Source: CAD feature listing. Evaluate the final solid. Frame: model axes, mm. A direction names the side the tool comes from. Round coordinates to 2 decimals unless told otherwise and drop trailing zeros. Order: outer loops, then holes, each group sorted by start corner. A loop starts at its lowest first (then second) coordinate and runs counter-clockwise, first axis right, second up. Notation, with made-up numbers: (3.25, -6) - (29.25, -6) arc R25 ccw to (29.25, 33) - close; hole circle Ø9 at (45, 35). An arc over 180 degrees is marked (long way). Use one line per item in the form item = value. Start each with the question number.
Q1. Ray query, line 1 (Z direction, x = -57.5, y = 9.25); line 2 (X direction, y = 5.25, z = 57.15); line 3 (X direction, y = -0.25, z = -63.5). Return the intervals inside material, ascending. Write a range as [from, to].
Q2. Draft query along X for faces 5 (the flat face through (-54.098, 19, 83)), 6 (the flat face through (53.15, 4, -1)), 7 (the flat face through (-57, 8, 1)), 8 (the flat face through (41, 17.05, -79)). Return one class per face: released by +X, released by -X, zero draft, split by the parting line, or undercut.
Q3. Cut plane B-B, the plane x = -18. Return the cut outline in (y, z).
Q4. Cut plane C-C, the plane y = 5.5. Give the number of separate pieces and of enclosed holes in the cut face, and give its area (3 significant figures).
Q5. Cut plane A-A, the plane z = 45. Return the cut outline in (x, y).
Q6. Set-up query: faces 1 (the flat face through (41.734, 5.448, -63.204)), 2 (the flat face through (-37.263, 19.022, -87.737)), 3 (the flat face through (27, 19, 72.2)), 4 (the flat face through (-61, 10, -57)). Return all of +Z, -Z, +X, -X, +Y, -Y with unobstructed straight access to the full face (end or side cutting, diameter ignored); none if empty.
Q7. Pin query (flat end, axial travel): pin 1 Ø17.5 at (x, z) = (54.5, 56.5) entering from +Y; pin 2 Ø6.5 at (x, y) = (26, 14) entering from -Z; pin 3 Ø1 at (y, z) = (15.5, 57.5) entering from -X; pin 4 Ø1.5 at (x, y) = (44.5, 9) entering from -Z. Return the tip coordinate at first contact, or that it passes through.
from build123d import *

# Parameters (mm, degrees)
BOSS_EXTRUDE1_DEPTH            = 8
BOSS_EXTRUDE2_DEPTH            = 2
BOSS_EXTRUDE3_DEPTH            = 9.05
SKETCH4_R                      = 2.25
BOSS_EXTRUDE4_DEPTH            = 4
CUT_EXTRUDE1_REACH             = 89.395
SKETCH5_W                      = 12.364675298
SKETCH5_H                      = 8
CUT_EXTRUDE1_DIRECTION_2_DEPTH = 88.395228364
CUT_EXTRUDE2_DEPTH             = 9.171573
CUT_EXTRUDE3_REACH             = 115.505
SKETCH8_W                      = 3.39411255
SKETCH8_H                      = 9.05
CUT_EXTRUDE3_DIRECTION_2_REACH = 115.505
BOSS_EXTRUDE5_DEPTH            = 16.456854
CUT_EXTRUDE4_DEPTH             = 114.504844196
SKETCH12_R                     = 3.6
CUT_EXTRUDE5_DEPTH             = 114.645358602
BOSS_EXTRUDE6_START            = 2
SKETCH13_W                     = 16
SKETCH13_H                     = 16
SKETCH13_R                     = 3.6
BOSS_EXTRUDE6_DEPTH            = 2
CUT_EXTRUDE6_REACH             = 182.475
CUT_EXTRUDE6_DIRECTION_2_DEPTH = 15


with BuildPart() as part:
    # Sketch1 → Boss-Extrude1 (new body)
    with BuildSketch(Plane(origin=(0, 0, 0), x_dir=(1, 0, 0), z_dir=(0, 1, 0))):
        Polygon((-53.15, 0), (-61.15, 0), (-61.15, -49.15), (-65.15, -49.15), (-65.15, -65.15), (-57.635281374, -65.15), (-32.585281374, -90.2), (0, -90.2), (0, -82.2), (-20.1, -82.2), (-20.1, -77.4), (-34.071572875, -77.4), (-39.3, -72.171572875), (-39.3, -58.2), (-49.15, -58.2), (-49.15, -49.15), (-53.15, -49.15), align=None)
    extrude(amount=BOSS_EXTRUDE1_DEPTH)

    # Sketch2 → Boss-Extrude2 (add)
    with BuildSketch(Plane.XZ):
        Polygon((-49.15, 58.2), (-49.15, 49.15), (-65.15, 49.15), (-65.15, 65.15), (-49.15, 65.15), align=None)
    extrude(amount=BOSS_EXTRUDE2_DEPTH)

    # Sketch3 → Boss-Extrude3 (add)
    with BuildSketch(Plane(origin=(0, 8, 0), x_dir=(1, 0, 0), z_dir=(0, 1, 0))):
        Polygon((-39.3, -58.2), (-45.3, -58.2), (-45.3, -74.656854249), (-36.556854249, -83.4), (-20.1, -83.4), (-20.1, -77.4), (-34.071572875, -77.4), (-39.3, -72.171572875), align=None)
    extrude(amount=BOSS_EXTRUDE3_DEPTH)

    # Sketch4 → Boss-Extrude4 (add)
    with BuildSketch(Plane(origin=(0, 17.05, 0), x_dir=(1, 0, 0), z_dir=(0, 1, 0))):
        Polygon((-45.3, -58.2), (-34.1, -58.2), (-34.1, -72.2), (-20.1, -72.2), (-20.1, -83.4), (-32.925631329, -83.4), (-41.723475836, -92.197844507), (-48.972213178, -92.197844507), (-54.097844507, -87.072213178), (-54.097844507, -79.823475836), (-45.3, -71.025631329), align=None)
        with Locations(Location((-45.347844507, -83.447844507, 0), (0, 0, 270))):
            Circle(SKETCH4_R, mode=Mode.SUBTRACT)
    extrude(amount=BOSS_EXTRUDE4_DEPTH)

    # Sketch5 → Cut-Extrude1 (cut, up to next)
    with BuildSketch(Plane(origin=(-59.978427125, 0, 59.978427125), x_dir=(0.7071067811865475, 0, 0.7071067811865477), z_dir=(-0.7071067811865477, 0, 0.7071067811865475)), mode=Mode.PRIVATE) as cut_extrude1_sk1:
        with Locations((26.940768363, 13.05)):
            Rectangle(SKETCH5_W, SKETCH5_H)
    cut_extrude1_tool1 = extrude(cut_extrude1_sk1.sketch, amount=-CUT_EXTRUDE1_REACH, mode=Mode.PRIVATE) & part.part
    add(cut_extrude1_tool1.solids().sort_by_distance((-40.928427, 13.05, 79.028427))[0], mode=Mode.SUBTRACT)

    # Sketch5 → Cut-Extrude1 direction 2 (cut)
    with BuildSketch(Plane(origin=(-59.978427125, 0, 59.978427125), x_dir=(0.7071067811865475, 0, 0.7071067811865477), z_dir=(-0.7071067811865477, 0, 0.7071067811865475))):
        with Locations((26.940768363, 13.05)):
            Rectangle(SKETCH5_W, SKETCH5_H)
    extrude(amount=CUT_EXTRUDE1_DIRECTION_2_DEPTH, mode=Mode.SUBTRACT)

    # Sketch6 → Cut-Extrude2 (cut)
    with BuildSketch(Plane(origin=(-20.1, 0, 0), x_dir=(0, 0, -1), z_dir=(1, 0, 0))):
        Polygon((-82.2, 0), (-77.4, 11.05), (-77.4, 0), align=None)
    cut_extrude2 = extrude(amount=-CUT_EXTRUDE2_DEPTH, mode=Mode.SUBTRACT)

    # Mirror1: Cut-Extrude2 across plane
    add(cut_extrude2.mirror(Plane(origin=(19.05, 0, 19.05), x_dir=(-0.7071067811865477, 0, 0.7071067811865474), z_dir=(0.7071067811865476, 0, 0.7071067811865476))), mode=Mode.SUBTRACT)

    # Cut-Extrude3: up to this face of the body (flat: up to its plane)
    cut_extrude3_end = Plane(part.part.faces().sort_by_distance((-41.7, 5.525, 62.7857865))[0])
    # Sketch8 → Cut-Extrude3 (cut, up to the picked face)
    with BuildSketch(Plane(origin=(19.05, 0, 19.05), x_dir=(0.7071067811865476, 0, -0.7071067811865476), z_dir=(0.7071067811865476, 0, 0.7071067811865476)), mode=Mode.PRIVATE) as cut_extrude3_sk1:
        with Locations((-77.125248815, 4.525)):
            Rectangle(SKETCH8_W, SKETCH8_H)
    cut_extrude3_tool1 = split(extrude(cut_extrude3_sk1.sketch, amount=-CUT_EXTRUDE3_REACH, mode=Mode.PRIVATE), bisect_by=cut_extrude3_end, keep=Keep.BOTH, mode=Mode.PRIVATE)
    add(cut_extrude3_tool1.solids().sort_by(Axis((-35.485786, 4.525, 73.585786), (-0.7071067811865476, 0, -0.7071067811865476)))[0], mode=Mode.SUBTRACT)

    # Cut-Extrude3 direction 2: up to this face of the body (flat: up to its plane)
    cut_extrude3_direction_2_end = Plane(part.part.faces().sort_by_distance((-24.6857865, 5.525, 79.8))[0])
    # Sketch8 → Cut-Extrude3 direction 2 (cut, up to the picked face)
    with BuildSketch(Plane(origin=(19.05, 0, 19.05), x_dir=(0.7071067811865476, 0, -0.7071067811865476), z_dir=(0.7071067811865476, 0, 0.7071067811865476)), mode=Mode.PRIVATE) as cut_extrude3_direction_2_sk1:
        with Locations((-77.125248815, 4.525)):
            Rectangle(SKETCH8_W, SKETCH8_H)
    cut_extrude3_direction_2_tool1 = split(extrude(cut_extrude3_direction_2_sk1.sketch, amount=CUT_EXTRUDE3_DIRECTION_2_REACH, mode=Mode.PRIVATE), bisect_by=cut_extrude3_direction_2_end, keep=Keep.BOTH, mode=Mode.PRIVATE)
    add(cut_extrude3_direction_2_tool1.solids().sort_by(Axis((-35.485786, 4.525, 73.585786), (0.7071067811865476, 0, 0.7071067811865476)))[0], mode=Mode.SUBTRACT)

    # Sketch10 → Boss-Extrude5 (add)
    with BuildSketch(Plane(origin=(-20.1, 0, 0), x_dir=(0, 0, -1), z_dir=(1, 0, 0))):
        Polygon((-83.4, 12.296887645), (-85.26652133, 8), (-83.4, 8), align=None)
    boss_extrude5 = extrude(amount=-BOSS_EXTRUDE5_DEPTH)

    # Sketch11 → Cut-Extrude4 (cut, through all)
    with BuildSketch(Plane(origin=(19.05, 0, 19.05), x_dir=(0.7071067811865476, 0, -0.7071067811865476), z_dir=(0.7071067811865476, 0, 0.7071067811865476))):
        Polygon((-84.82230509, 12.296887645), (-86.142134979, 8), (-84.82230509, 8), align=None)
    cut_extrude4 = extrude(amount=CUT_EXTRUDE4_DEPTH, mode=Mode.SUBTRACT)

    # Mirror2: Boss-Extrude5, Cut-Extrude4 across plane
    add(boss_extrude5.mirror(Plane(origin=(19.05, 0, 19.05), x_dir=(-0.7071067811865477, 0, 0.7071067811865474), z_dir=(0.7071067811865476, 0, 0.7071067811865476))))
    add(cut_extrude4.mirror(Plane(origin=(19.05, 0, 19.05), x_dir=(-0.7071067811865477, 0, 0.7071067811865474), z_dir=(0.7071067811865476, 0, 0.7071067811865476))), mode=Mode.SUBTRACT)

    # Sketch12 → Cut-Extrude5 (cut, through all)
    with BuildSketch(Plane(origin=(0, 8, 0), x_dir=(1, 0, 0), z_dir=(0, 1, 0))):
        with Locations(Location((-57.15, -57.15, 0), (0, 0, 270))):
            Circle(SKETCH12_R)
    extrude(amount=-CUT_EXTRUDE5_DEPTH, mode=Mode.SUBTRACT)

    # Mirror3: part across plane


with BuildPart() as part_1:
    add(part.part)
    add(part.part.mirror(Plane(origin=(-53.15, 8, 0), x_dir=(1, 0, 0), z_dir=(0, 0, 1))))

    # Mirror4: part across plane


with BuildPart() as part_2:
    add(part_1.part)
    add(part_1.part.mirror(Plane(origin=(0, 8, -90.2), x_dir=(0, 0, 1), z_dir=(-1, 0, 0))))

    # Sketch13 → Boss-Extrude6 (add)
    # profile 1 of 4: a face of its own
    with BuildSketch(Plane(origin=(0, 8, 0), x_dir=(1, 0, 0), z_dir=(0, 1, 0)).offset(BOSS_EXTRUDE6_START)):
        with Locations((-57.15, 57.15)):
            Rectangle(SKETCH13_W, SKETCH13_H)
        with Locations(Location((-57.15, 57.15, 0), (0, 0, 90))):
            Circle(SKETCH13_R, mode=Mode.SUBTRACT)
    # profile 2 of 4: a face of its own
    with BuildSketch(Plane(origin=(0, 8, 0), x_dir=(1, 0, 0), z_dir=(0, 1, 0)).offset(BOSS_EXTRUDE6_START)):
        with Locations((-57.15, -57.15)):
            Rectangle(SKETCH13_W, SKETCH13_H)
        with Locations(Location((-57.15, -57.15, 0), (0, 0, 270))):
            Circle(SKETCH13_R, mode=Mode.SUBTRACT)
    # profile 3 of 4: a face of its own
    with BuildSketch(Plane(origin=(0, 8, 0), x_dir=(1, 0, 0), z_dir=(0, 1, 0)).offset(BOSS_EXTRUDE6_START)):
        with Locations((57.15, -57.15)):
            Rectangle(SKETCH13_W, SKETCH13_H)
        with Locations(Location((57.15, -57.15, 0), (0, 0, 270))):
            Circle(SKETCH13_R, mode=Mode.SUBTRACT)
    # profile 4 of 4: a face of its own
    with BuildSketch(Plane(origin=(0, 8, 0), x_dir=(1, 0, 0), z_dir=(0, 1, 0)).offset(BOSS_EXTRUDE6_START)):
        with Locations((57.15, 57.15)):
            Rectangle(SKETCH13_W, SKETCH13_H)
        with Locations(Location((57.15, 57.15, 0), (0, 0, 90))):
            Circle(SKETCH13_R, mode=Mode.SUBTRACT)
    extrude(amount=-BOSS_EXTRUDE6_DEPTH)

    # Cut-Extrude6: up to this face of the body (flat: up to its plane)
    cut_extrude6_end = Plane(part_2.part.faces().sort_by_distance((25.508916271, 13.892566464, 77.4))[0])
    # Sketch14 → Cut-Extrude6 (cut, up to the picked face)
    with BuildSketch(Plane(origin=(0, 0, 74.785786438), x_dir=(-1, 0, 0), z_dir=(0, 0, -1)), mode=Mode.PRIVATE) as cut_extrude6_sk1:
        with BuildLine():
            Line((-38.891815428, 9.05), (-29.271572875, 9.05))
            Line((-29.271572875, 9.05), (-29.271572875, 0))
            Line((-29.271572875, 0), (-37.428466034, 0))
            ThreePointArc((-37.428466034, 0), (-38.292196947, 4.503647029), (-38.891815428, 9.05))
        make_face()
    cut_extrude6_tool1 = split(extrude(cut_extrude6_sk1.sketch, amount=-CUT_EXTRUDE6_REACH, mode=Mode.PRIVATE), bisect_by=cut_extrude6_end, keep=Keep.BOTH, mode=Mode.PRIVATE)
    add(cut_extrude6_tool1.solids().sort_by(Axis((33.771048, 4.647825, 74.785786), (0, 0, 1)))[0], mode=Mode.SUBTRACT)

    # Sketch14 → Cut-Extrude6 direction 2 (cut)
    with BuildSketch(Plane(origin=(0, 0, 74.785786438), x_dir=(-1, 0, 0), z_dir=(0, 0, -1))):
        with BuildLine():
            Line((-38.891815428, 9.05), (-29.271572875, 9.05))
            Line((-29.271572875, 9.05), (-29.271572875, 0))
            Line((-29.271572875, 0), (-37.428466034, 0))
            ThreePointArc((-37.428466034, 0), (-38.292196947, 4.503647029), (-38.891815428, 9.05))
        make_face()
    extrude(amount=CUT_EXTRUDE6_DIRECTION_2_DEPTH, mode=Mode.SUBTRACT)


solid = part_2.part
Completed:
q1.line_1 = [-65.15, -60.73], [-53.57, -49.15], [49.15, 53.57], [60.73, 65.15]
q1.line_2 = [-65.15, -60.75], [-53.55, -49.15], [49.15, 53.55], [60.75, 65.15]
q1.line_3 = [-65.15, -49.15], [49.15, 65.15]
q2.face_5 = released by -X
q2.face_6 = undercut
q2.face_7 = zero draft
q2.face_8 = undercut
q3.outline = (0, -90.2) - (8, -90.2) - (8, -82.2) - (0, -82.2) - close; (0, 82.2) - (8, 82.2) - (8, 90.2) - (0, 90.2) - close
q4.separate_pieces = 1
q4.enclosed_holes = 5
q4.area = 4,720 mm2
q5.outline = (-61.15, 0) - (-53.15, 0) - (-53.15, 8) - (-61.15, 8) - close; (53.15, 0) - (61.15, 0) - (61.15, 8) - (53.15, 8) - close
q6.face_1 = -Y
q6.face_2 = -Z, +Y
q6.face_3 = +Y, -Y
q6.face_4 = +Z, -Z, -X, +Y
q7.pin_1 = 10.88
q7.pin_2 = -84.07
q7.pin_3 = through
q7.pin_4 = -76.21
